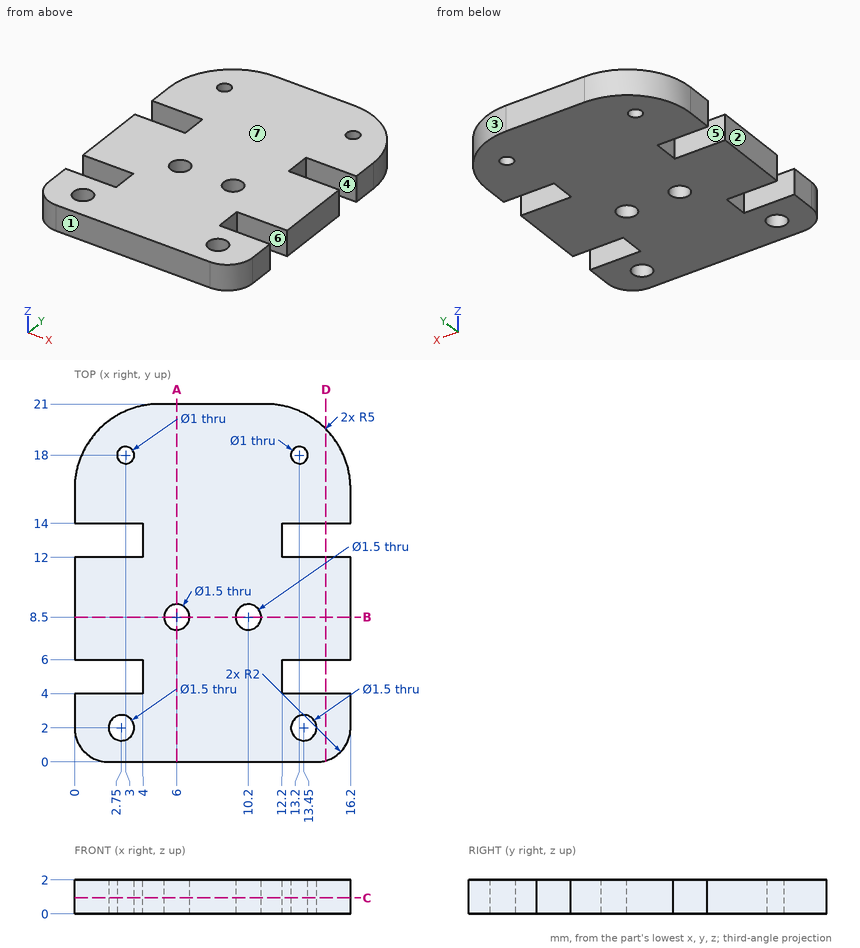
Answer from the drawing. Dimensions are ordinates in mm from the lowest x, y and z of the part. A direction names the side the tool comes from. Coordinates: 2 decimals unless noted, no trailing zeros. Order: outer loops, then holes, each group sorted by start corner. A loop starts at its lowest first (then second) coordinate and runs counter-clockwise, first axis right, second up. Notation, with made-up numbers: (86, 89.5) -> (94, 89.5) arc R13 ccw to (94, 105.5) -> close; hole circle Ø1 at (-22.75, -15). An arc over 180 degrees is marked (long way). Answer as a JSON object with one key per item and string values.
1) The mould has two halves that part along Y. Classify the marked faces 1, 2, 3 and 4: released by +Y, released by -Y, zero draft, split by the parting line, or undercut.
Model answer:
{"face 1": "released by -Y", "face 2": "zero draft", "face 3": "released by +Y", "face 4": "undercut"}
2) A cutting plane is placed at B-B, the plane y = 8.5. Determine the outline of the cut face in (x, z).
Model answer:
{"outline": "(0, 0) -> (5.25, 0) -> (5.25, 2) -> (0, 2) -> close; (6.75, 0) -> (9.45, 0) -> (9.45, 2) -> (6.75, 2) -> close; (10.95, 0) -> (16.2, 0) -> (16.2, 2) -> (10.95, 2) -> close"}
3) Each of these flat-tipped pins is pushed along its axis until it touches: pin 1 (2 mm diameter, centred on x = 6, y = 8.5, fed in from -Z); pin 2 (1 mm diameter, centred on y = 5, z = 0.5, fed in from +X); pin 3 (1 mm diameter, centred on x = 13.5, z = 2, fed in from +Y); pin 4 (1 mm diameter, centred on x = 15, z = 1, fed in from -Y). Where does it stop, or does it pass through?
Model answer:
{"pin 1": "stops at z = 0", "pin 2": "stops at x = 12.2", "pin 3": "stops at y = 20.66", "pin 4": "stops at y = 0.02"}
4) A tool of negligible diameter and unlimited length cuts with its end or side. For the marked faces 5, 6 and 7, from which of +Z, -Z, +X, -X, +Y, -Y can it reach the whole face along a straight path? Write none if from no direction.
Model answer:
{"face 5": "+Z, -Z, -X", "face 6": "+Z, -Z, +X", "face 7": "+Z, +X, -X, +Y, -Y"}
5) A cutting plane is placed at D-D, the plane x = 14.75. Determine the outline of the cut face in (y, z).
Model answer:
{"outline": "(0.08, 0) -> (4, 0) -> (4, 2) -> (0.08, 2) -> close; (6, 0) -> (12, 0) -> (12, 2) -> (6, 2) -> close; (14, 0) -> (19.52, 0) -> (19.52, 2) -> (14, 2) -> close"}
6) A cutting plane is placed at C-C, the plane z = 0.95. State how many separate pieces and enclosed holes the cut face has, plus the area to 3 significant figures.
Model answer:
{"separate pieces": "1", "enclosed holes": "6", "area": "287 mm²"}
7) Consider line 1 along Y through (x, z) = (10.2, 1.35); line 2 along Y through (x, z) = (13.5, 1); line 3 along Y through (x, z) = (15, 1.5). Determine where each line is inside the solid, lowest interval first. Write a range as from..to.
Model answer:
{"line 1": "y = 0..7.75, 9.25..21", "line 2": "y = 0..1.25, 2.75..4, 6..12, 14..17.6, 18.4..20.44", "line 3": "y = 0.17..4, 6..12, 14..19.25"}
8) A cutting plane is placed at A-A, the plane x = 6. Determine the outline of the cut face in (y, z), plus the area to 3 significant figures.
Model answer:
{"outline": "(0, 0) -> (7.75, 0) -> (7.75, 2) -> (0, 2) -> close; (9.25, 0) -> (21, 0) -> (21, 2) -> (9.25, 2) -> close", "area": "39.0 mm²"}
